The model under review builds one solid part; all positions refer to its coordinate system, in mm. A direction names the side the tool comes from. Round coordinates to 2 decimals unless told otherwise and drop trailing zeros. Loops run counter-clockwise (first coordinate to the right, second up) from the corner with the lowest first, then second, coordinate; pieces in that order, holes last. Notation, with made-up numbers: M 63,10 L 102,10 A10 cw 102,28 Z; hole C 60,-37 d11. An arc over 180 degrees is marked long. Answer as a JSON object with one key per item and string values. Group by question number.
Item 1: Tool access review of faces 1 (the face through (27.92, 3, -25)), 2 (the face through (27.92, 3, 25)), 3 (the face through (30, 3, -5)), 4 (the face through (0, 3, -21.5)), 5 (the face through (-30, 3, -5)): name each direction out of +Z, -Z, +X, -X, +Y, -Y from which nothing blocks a thin tool from reaching the whole face with its end or side.
Item 2: Consider section A-A (x = -17). Give the boundary of the cut face in (y, z).
Item 3: To check wall thickness, follow line 1 (Z direction, x = -17, y = 1.45); line 2 (X direction, y = 1.4, z = -13.5); line 3 (Z direction, x = 8, y = 0.45). State the ranges of each line that lie inside material, in increasing order.
Item 4: Consider section B-B (z = 8.5). Give the boundary of the cut face in (x, y).
Item 5: Consider section C-C (x = -26.5). Give the boundary of the cut face in (y, z).
Item 6: Insertion check: P1, Ø2.5, axis at x = 30, y = 2.5, coming from the -Z side; P2, Ø2.5, axis at x = -30.5, y = 2, coming from the +Z side; P3, Ø2.5, axis at x = -30, y = 1.5, coming from the -Z side. Each pin has a flat end and moves straight along its axis. Give the tip position at first contact, or say it passes through.
Item 7: Consider section D-D (y = 3.7). State how many separate pieces and enclosed holes the cut face has, and give its area (3 significant figures).
Item 8: The part is to be moulded in two halves that separate along Z. For faces 6 (the face through (-30, 3, -50)), 7 (the face through (0, 3, 23.5)), 8 (the face through (-33, 3, -45)), say which applies: +Z half, -Z half, draft (parallel to the pull), parting line (faces both ways), or undercut.
```python
from build123d import *

# Parameters (mm, degrees)
SKETCH1_W           = 55.84
SKETCH1_H           = 60
SKETCH1_W_2         = 45
SKETCH1_H_2         = 45
BOSS_EXTRUDE1_DEPTH = 5.08
SKETCH2_W           = 5.08
SKETCH2_H           = 15
BOSS_EXTRUDE2_DEPTH = 5.08
SKETCH3_R           = 7.5
BOSS_EXTRUDE3_DEPTH = 5.08
FILLET1_R           = 20
SKETCH4_W           = 5.08
SKETCH4_H           = 12
CUT_EXTRUDE1_DEPTH  = 6.08


with BuildPart() as part:
    # Sketch1 → Boss-Extrude1 (new body)
    with BuildSketch(Plane(origin=(0, 0, 0), x_dir=(1, 0, 0), z_dir=(0, 1, 0))):
        Rectangle(SKETCH1_W, SKETCH1_H)
        with Locations((0.5, -1)):
            Rectangle(SKETCH1_W_2, SKETCH1_H_2, mode=Mode.SUBTRACT)
    extrude(amount=BOSS_EXTRUDE1_DEPTH)

    # Sketch2 → Boss-Extrude2 (add)
    with BuildSketch(Plane(origin=(0, 5.08, 0), x_dir=(1, 0, 0), z_dir=(0, 1, 0))):
        with Locations((-30.46, -12.5)):
            Rectangle(SKETCH2_W, SKETCH2_H)
        with Locations((30.46, -12.5)):
            Rectangle(SKETCH2_W, SKETCH2_H)
        with Locations((-30.46, 12.5)):
            Rectangle(SKETCH2_W, SKETCH2_H)
        with Locations((30.46, 12.5)):
            Rectangle(SKETCH2_W, SKETCH2_H)
    extrude(amount=-BOSS_EXTRUDE2_DEPTH)

    # Sketch3 → Boss-Extrude3 (add)
    with BuildSketch(Plane(origin=(0, 5.08, 0), x_dir=(1, 0, 0), z_dir=(0, 1, 0))):
        Polygon((-7.5, 30), (7.5, 30), (7.5, 40), (7.5, 62), (-33, 62), (-33, 40), (-7.5, 40), align=None)
        with Locations((-17, 51)):
            Circle(SKETCH3_R, mode=Mode.SUBTRACT)
    extrude(amount=-BOSS_EXTRUDE3_DEPTH)

    # Fillet1
    fillet1_edges = [part.edges().sort_by_distance(p)[0] for p in [
        (7.5, 2.54, -62),
    ]]
    fillet(fillet1_edges, radius=FILLET1_R)

    # Sketch4 → Cut-Extrude1 (cut, through all)
    with BuildSketch(Plane(origin=(0, 5.08, 0), x_dir=(1, 0, 0), z_dir=(0, 1, 0))):
        with Locations((-30.46, 56)):
            Rectangle(SKETCH4_W, SKETCH4_H)
    extrude(amount=-CUT_EXTRUDE1_DEPTH, mode=Mode.SUBTRACT)


solid = part.part
```
Geometry results:
{
 "1": {"face 1": "-Z, +X, +Y, -Y", "face 2": "+Z, +X, +Y, -Y", "face 3": "+X, +Y, -Y", "face 4": "+Y, -Y", "face 5": "-X, +Y, -Y"},
 "2": {"outline": "M 0,-62 L 5.08,-62 L 5.08,-58.5 L 0,-58.5 Z; M 0,-43.5 L 5.08,-43.5 L 5.08,-40 L 0,-40 Z; M 0,-30 L 5.08,-30 L 5.08,-21.5 L 0,-21.5 Z; M 0,23.5 L 5.08,23.5 L 5.08,30 L 0,30 Z"},
 "3": {"line 1": "z = -62 to -58.5, -43.5 to -40, -30 to -21.5, 23.5 to 30", "line 2": "x = -33 to -22, 23 to 33", "line 3": "z = -30 to -21.5, 23.5 to 30"},
 "4": {"outline": "M -33,0 L -22,0 L -22,5.08 L -33,5.08 Z; M 23,0 L 33,0 L 33,5.08 L 23,5.08 Z"},
 "5": {"outline": "M 0,-62 L 5.08,-62 L 5.08,-40 L 0,-40 Z; M 0,-30 L 5.08,-30 L 5.08,30 L 0,30 Z"},
 "6": {"P1": "stops at z = -20", "P2": "stops at z = 20", "P3": "stops at z = -50"},
 "7": {"separate pieces": "1", "enclosed holes": "2", "area": "2,350 mm^2"},
 "8": {"face 6": "-Z half", "face 7": "undercut", "face 8": "draft"}
}
